Check sheet for the modelled part. Datum: model origin and axes. Units: mm. Round coordinates to 2 decimals unless told otherwise and drop trailing zeros. Loops run counter-clockwise (first coordinate to the right, second up) from the corner with the lowest first, then second, coordinate; pieces in that order, holes last. Notation, with made-up numbers: (7, 57.5) - (66, 57.5) arc R24 cw to (66, 82.5) - close; hole circle Ø11 at (39.5, 31.5). An arc over 180 degrees is marked (long way). Put each result on its own line as item: value. Start each with the question number.
Item 1: Gauge pin test, flat ends, axial feed: pin 1 Ø3 at (x, z) = (3, 26) entering from -Y; pin 2 Ø2 at (x, z) = (2, -7) entering from +Y; pin 3 Ø2.5 at (y, z) = (-19, -53.29) entering from +X; pin 4 Ø1.8 at (x, y) = (3.5, -57) entering from -Z. Record the tip position at first contact, or that the pin passes through.
Item 2: Section check C-C, the plane z = 1.5. Record the cut outline in (x, y), and give its area (3 significant figures).
Item 3: Section check A-A, the plane y = 41. Record the cut outline in (x, z), and give its area (3 significant figures).
Item 4: Section check B-B, the plane x = 3.15. Give the number of separate pieces and of enclosed holes in the cut face, and give its area (3 significant figures).
Item 5: Material ranges on line 1 along Y through (x, z) = (4.7, 38.71); line 2 along Z through (x, y) = (2.75, -79); line 3 along Y through (x, z) = (2.4, -51.5), recorded low to high.
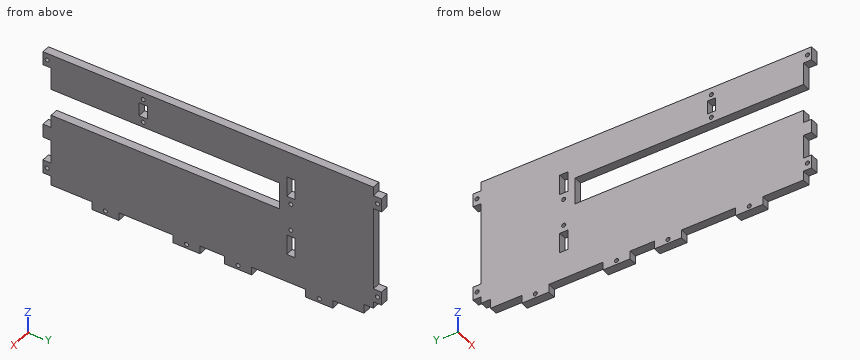
from build123d import *

# Parameters (mm, degrees)
ESQUISSE1_W             = 100.58
ESQUISSE1_H             = 238
ESQUISSE1_W_2           = 10
ESQUISSE1_H_2           = 6
ESQUISSE1_W_3           = 15
BOSS_EXTRU_1_DEPTH      = 6
ESQUISSE3_W             = 10
ESQUISSE3_H             = 6
ESQUISSE3_W_2           = 6
ESQUISSE3_H_2           = 20
BOSS_EXTRU_5_DEPTH      = 6
ESQUISSE6_W             = 20
ESQUISSE6_H             = 168.59
ENL_V_MAT_EXTRU_2_DEPTH = 6
ESQUISSE7_W             = 6.88
ESQUISSE7_H             = 7
ENL_V_MAT_EXTRU_3_DEPTH = 6
ESQUISSE8_R             = 1.5
ENL_V_MAT_EXTRU_4_DEPTH = 6


with BuildPart() as part:
    # Esquisse1 → Boss.-Extru.1 (new body)
    with BuildSketch(Plane(origin=(0, 0, 0), x_dir=(0, 0, -1), z_dir=(1, 0, 0))):
        Rectangle(ESQUISSE1_W, ESQUISSE1_H)
        with Locations((-36.29, -51)):
            Rectangle(ESQUISSE1_W_2, ESQUISSE1_H_2, mode=Mode.SUBTRACT)
        with Locations((-23.295, 58)):
            Rectangle(ESQUISSE1_W_3, ESQUISSE1_H_2, mode=Mode.SUBTRACT)
        with Locations((21.705, 58)):
            Rectangle(ESQUISSE1_W_3, ESQUISSE1_H_2, mode=Mode.SUBTRACT)
    extrude(amount=BOSS_EXTRU_1_DEPTH)

    # Esquisse3 → Boss.-Extru.5 (add)
    with BuildSketch(Plane(origin=(6, 0, 0), x_dir=(0, 0, -1), z_dir=(1, 0, 0))):
        with Locations((-45.29, -122)):
            Rectangle(ESQUISSE3_W, ESQUISSE3_H)
        with Locations((38.41, -122)):
            Rectangle(ESQUISSE3_W, ESQUISSE3_H)
        with Locations((53.29, 19)):
            Rectangle(ESQUISSE3_W_2, ESQUISSE3_H_2)
        with Locations((53.29, 79)):
            Rectangle(ESQUISSE3_W_2, ESQUISSE3_H_2)
        with Locations((53.29, -79)):
            Rectangle(ESQUISSE3_W_2, ESQUISSE3_H_2)
        with Locations((53.29, -19)):
            Rectangle(ESQUISSE3_W_2, ESQUISSE3_H_2)
        with Locations((10.79, -122)):
            Rectangle(ESQUISSE3_W, ESQUISSE3_H)
        with Locations((33.41, 122)):
            Rectangle(ESQUISSE3_W, ESQUISSE3_H)
        with Locations((-38.71, 122)):
            Rectangle(ESQUISSE3_W, ESQUISSE3_H)
    extrude(amount=-BOSS_EXTRU_5_DEPTH)

    # Esquisse6 → Enlèv. mat.-Extru.2 (cut)
    with BuildSketch(Plane(origin=(6, 0, 0), x_dir=(0, 0, -1), z_dir=(1, 0, 0))):
        with Locations((-13.71, -34.705)):
            Rectangle(ESQUISSE6_W, ESQUISSE6_H)
    extrude(amount=-ENL_V_MAT_EXTRU_2_DEPTH, mode=Mode.SUBTRACT)

    # Esquisse7 → Enlèv. mat.-Extru.3 (cut)
    with BuildSketch(Plane.ZY):
        with Locations((-46.85, 115.5)):
            Rectangle(ESQUISSE7_W, ESQUISSE7_H)
    extrude(amount=-ENL_V_MAT_EXTRU_3_DEPTH, mode=Mode.SUBTRACT)

    # Esquisse8 → Enlèv. mat.-Extru.4 (cut)
    with BuildSketch(Plane.ZY):
        with Locations((-9.205, 58)):
            Circle(ESQUISSE8_R)
        with Locations((10.795, 58)):
            Circle(ESQUISSE8_R)
        with Locations((27.5, -51)):
            Circle(ESQUISSE8_R)
        with Locations((45.08, -51)):
            Circle(ESQUISSE8_R)
        with Locations((38.71, 122)):
            Circle(ESQUISSE8_R)
        with Locations((-33.41, 122)):
            Circle(ESQUISSE8_R)
        with Locations((45.29, -122)):
            Circle(ESQUISSE8_R)
        with Locations((-53.29, 79)):
            Circle(ESQUISSE8_R)
        with Locations((-38.41, -122)):
            Circle(ESQUISSE8_R)
        with Locations((-53.29, 19)):
            Circle(ESQUISSE8_R)
        with Locations((-53.29, -79)):
            Circle(ESQUISSE8_R)
        with Locations((-53.29, -19)):
            Circle(ESQUISSE8_R)
    extrude(amount=-ENL_V_MAT_EXTRU_4_DEPTH, mode=Mode.SUBTRACT)


solid = part.part
Check result:
1. pin 1: y = -119
1. pin 2: y = 119
1. pin 3: through
1. pin 4: z = -50.29
2. outline: (0, -119) - (6, -119) - (6, 119) - (0, 119) - close
2. area: 1,430 mm²
3. outline: (0, -50.29) - (6, -50.29) - (6, 3.71) - (0, 3.71) - close; (0, 23.71) - (6, 23.71) - (6, 50.29) - (0, 50.29) - close
3. area: 483 mm²
4. separate pieces: 1
4. enclosed holes: 15
4. area: 21,000 mm²
5. line 1: -119 to -54, -48 to 120.5, 123.5 to 125
5. line 2: -56.29 to -54.79, -51.79 to 3.71, 23.71 to 50.29
5. line 3: -89 to -69, -29 to -9, 9 to 29, 69 to 89
